Could you check a few things on this model? Use its own coordinates, in mm. A direction names the side the tool comes from. Give positions to 0.01 mm unless a question says otherwise; leave off trailing zeros. Loops run counter-clockwise (first coordinate to the right, second up) from the corner with the lowest first, then second, coordinate; pieces in that order, holes last. Notation, with made-up numbers: (84, -7) - (109, -7) arc R23 cw to (109, 1) - close; hole circle Ø11 at (-8.5, 3). An arc over 180 degrees is marked (long way). Write each question's results on one line, items separated by ' | '. Start each with the question number.
(1) If we mould it in two halves opening along Y, with no side actions, what happens to faces 4 (the face through (-103.158, -102, 19)), 5 (the face through (-101.73, -133.28, 19.72)), 6 (the face through (-35.66, -73.21, 18.24))? For each: released by +Y, released by -Y, zero draft, split by the parting line, or undercut.
(2) Suppose I cut it at C-C (y = -117.5). Please give me the cut outline in (x, z).
(3) On a 3-axis mill with a long thin cutter (end or side, diameter ignored), from which of +Z, -Z, +X, -X, +Y, -Y can I reach the whole of each face in a straight line? I mean faces 1 (the face through (-32.679, -116.549, 56.375)), 2 (the face through (-100.158, -102, 54)), 3 (the face through (-98.65, -130.36, 18.24)). Say none if no direction works.
(4) Suppose I cut it at B-B (x = -44). Please give me the cut outline in (y, z).
(5) I need wall thicknesses on line 1 (Y direction, x = -71.5, z = 5.5); line 2 (X direction, y = -122.5, z = 21); line 3 (Z direction, x = -89, y = -116). Which ranges of each line are inside material? Lowest first, please.
(6) For pin 1 (18 mm diameter, centred on y = -92.5, z = 55.5, fed in from -X); pin 2 (8 mm diameter, centred on x = -94, y = -85.5, fed in from +Z); pin 3 (1 mm diameter, centred on x = -47.5, y = -78.5, fed in from -Z); pin 4 (3.5 mm diameter, centred on x = -67.16, z = 15, fed in from -Y), each with a flat end and sliding along its axis, tell me the tip position at first contact or that it passes through.
(7) Suppose I cut it at A-A (z = 15). Please give me the cut outline in (x, y), and give its area (3 significant figures).
(8) Suppose I cut it at D-D (y = -81.5). Please give me the cut outline in (x, z), and give its area (3 significant figures).
from build123d import *

# Parameters (mm, degrees)
F1_DEPTH = 40
F3_DEPTH = 3
F5_DEPTH = 3
F7_DEPTH = 3
F9_D     = 3.1
F11_D    = 3.1


with BuildPart() as f1:
    # F0 (on Top) → F1 (new body)
    with BuildSketch(Plane.XY):
        with BuildLine():
            ThreePointArc((-98.1582802534, -68.7836479545), (-101.6938141593, -70.2481140485), (-103.1582802534, -73.7836479545))
            Line((-103.1582802534, -73.7836479545), (-103.1582802534, -129.7836479545))
            ThreePointArc((-103.1582802534, -129.7836479545), (-101.6938141593, -133.3191818604), (-98.1582802534, -134.7836479545))
            Line((-98.1582802534, -134.7836479545), (-36.1582802534, -134.7836479545))
            ThreePointArc((-36.1582802534, -134.7836479545), (-32.6227463475, -133.3191818604), (-31.1582802534, -129.7836479545))
            Line((-31.1582802534, -129.7836479545), (-31.1582802534, -73.7836479545))
            ThreePointArc((-31.1582802534, -73.7836479545), (-32.6227463475, -70.2481140485), (-36.1582802534, -68.7836479545))
            Line((-36.1582802534, -68.7836479545), (-98.1582802534, -68.7836479545))
        make_face()
        with BuildLine():
            ThreePointArc((-100.1582802534, -76.7836479545), (-98.6938141593, -73.2481140485), (-95.1582802534, -71.7836479545))
            Line((-95.1582802534, -71.7836479545), (-39.1582802534, -71.7836479545))
            ThreePointArc((-39.1582802534, -71.7836479545), (-35.6227463475, -73.2481140485), (-34.1582802534, -76.7836479545))
            Line((-34.1582802534, -76.7836479545), (-34.1582802534, -126.7836479545))
            ThreePointArc((-34.1582802534, -126.7836479545), (-35.6227463475, -130.3191818604), (-39.1582802534, -131.7836479545))
            Line((-39.1582802534, -131.7836479545), (-95.1582802534, -131.7836479545))
            ThreePointArc((-95.1582802534, -131.7836479545), (-98.6938141593, -130.3191818604), (-100.1582802534, -126.7836479545))
            Line((-100.1582802534, -126.7836479545), (-100.1582802534, -76.7836479545))
        make_face(mode=Mode.SUBTRACT)
    extrude(amount=F1_DEPTH)

    # F2 (on face) → F3 (join)
    with BuildSketch(Plane.YZ.offset(-100.1582802534)):
        with BuildLine():
            Line((-106.0236394745, 73.216013568), (-126.7836479545, 40))
            Line((-126.7836479545, 40), (-76.7836479545, 40))
            Line((-76.7836479545, 40), (-97.5436564344, 73.216013568))
            ThreePointArc((-97.5436564344, 73.216013568), (-101.7836479545, 75.5660188679), (-106.0236394745, 73.216013568))
        make_face()
    extrude(amount=-F3_DEPTH)

    # F4 (on face) → F5 (join)
    with BuildSketch(Plane(origin=(-34.1582802534, 0, 0), x_dir=(0, -1, 0), z_dir=(-1, 0, 0))):
        with BuildLine():
            Line((97.5436564344, 73.216013568), (76.7836479545, 40))
            Line((76.7836479545, 40), (80.8389559388, 40))
            Line((80.8389559388, 40), (126.7836479545, 40))
            Line((126.7836479545, 40), (106.0236394745, 73.216013568))
            ThreePointArc((106.0236394745, 73.216013568), (101.7836479545, 75.5660188679), (97.5436564344, 73.216013568))
        make_face()
    extrude(amount=-F5_DEPTH)

    # F6 (on face) → F7 (join)
    with BuildSketch(Plane.XY.offset(40)):
        with BuildLine():
            Line((-36.3776951637, -68.5804857016), (-98.3776951637, -68.5804857016))
            ThreePointArc((-98.3776951637, -68.5804857016), (-101.9132290697, -70.0449517956), (-103.3776951637, -73.5804857016))
            Line((-103.3776951637, -73.5804857016), (-103.3776951637, -129.5804857016))
            ThreePointArc((-103.3776951637, -129.5804857016), (-102.9290181233, -131.6506207979), (-101.6635114368, -133.349227059))
            ThreePointArc((-101.6635114368, -133.349227059), (-102.7694707676, -131.716759964), (-103.1582802534, -129.7836479545))
            Line((-103.1582802534, -129.7836479545), (-103.1582802534, -126.7836479545))
            Line((-103.1582802534, -126.7836479545), (-100.1582802534, -126.7836479545))
            ThreePointArc((-100.1582802534, -126.7836479545), (-98.6938141593, -130.3191818604), (-95.1582802534, -131.7836479545))
            Line((-95.1582802534, -131.7836479545), (-39.1582802534, -131.7836479545))
            ThreePointArc((-39.1582802534, -131.7836479545), (-35.6227463475, -130.3191818604), (-34.1582802534, -126.7836479545))
            Line((-34.1582802534, -126.7836479545), (-31.3776951637, -126.7836479545))
            Line((-31.3776951637, -126.7836479545), (-31.3776951637, -73.5804857016))
            ThreePointArc((-31.3776951637, -73.5804857016), (-32.8421612578, -70.0449517956), (-36.3776951637, -68.5804857016))
        make_face()
    extrude(amount=-F7_DEPTH)

    # F9 (through all)
    with Locations(Plane.YZ.offset(-31.1582802534)):
        with Locations((-101.7836479545, 70.5660188679)):
            Hole(F9_D / 2)

    # F11 (through all)
    with Locations(Plane.XZ.offset(134.7836479545)):
        with Locations((-67.1582802534, 15)):
            Hole(F11_D / 2)


solid = f1.part
Output values:
1) face 4: zero draft | face 5: released by -Y | face 6: undercut
2) outline: (-103.38, 37) - (-103.16, 37) - (-103.16, 0) - (-100.16, 0) - (-100.16, 37) - (-34.16, 37) - (-34.16, 0) - (-31.16, 0) - (-31.16, 54.85) - (-34.16, 54.85) - (-34.16, 40) - (-100.16, 40) - (-100.16, 54.85) - (-103.16, 54.85) - (-103.16, 40) - (-103.38, 40) - close
3) face 1: +Z, +X, -X, -Y | face 2: +Z, +Y, -Y | face 3: -Z
4) outline: (-134.78, 0) - (-131.78, 0) - (-131.78, 37) - (-71.78, 37) - (-71.78, 0) - (-68.78, 0) - (-68.78, 37) - (-68.58, 37) - (-68.58, 40) - (-134.78, 40) - close
5) line 1: -134.78 to -131.78, -71.78 to -68.78 | line 2: -103.16 to -100.16, -34.16 to -31.16 | line 3: 37 to 40
6) pin 1: x = -103.16 | pin 2: z = 40 | pin 3: z = 37 | pin 4: y = -134.78
7) outline: (-103.16, -129.78) arc R5 ccw to (-98.16, -134.78) - (-68.71, -134.78) - (-68.71, -131.78) - (-95.16, -131.78) arc R5 cw to (-100.16, -126.78) - (-100.16, -76.78) arc R5 cw to (-95.16, -71.78) - (-68.71, -71.78) - (-68.71, -68.78) - (-98.16, -68.78) arc R5 ccw to (-103.16, -73.78) - close; (-65.61, -134.78) - (-36.16, -134.78) arc R5 ccw to (-31.16, -129.78) - (-31.16, -73.78) arc R5 ccw to (-36.16, -68.78) - (-65.61, -68.78) - (-65.61, -71.78) - (-39.16, -71.78) arc R5 cw to (-34.16, -76.78) - (-34.16, -126.78) arc R5 cw to (-39.16, -131.78) - (-65.61, -131.78) - close | area: 773 mm2
8) outline: (-103.38, 37) - (-103.16, 37) - (-103.16, 0) - (-100.16, 0) - (-100.16, 37) - (-34.16, 37) - (-34.16, 0) - (-31.16, 0) - (-31.16, 47.55) - (-34.16, 47.55) - (-34.16, 40) - (-100.16, 40) - (-100.16, 47.55) - (-103.16, 47.55) - (-103.16, 40) - (-103.38, 40) - close | area: 484 mm2
